CAD build for the part. Positions are in the model's coordinates, mm. Face numbers are marked on the shaded views. Give positions to 0.01 mm unless a question says otherwise; leave off trailing zeros. Loops run counter-clockwise (first coordinate to the right, second up) from the corner with the lowest first, then second, coordinate; pieces in that order, holes last.
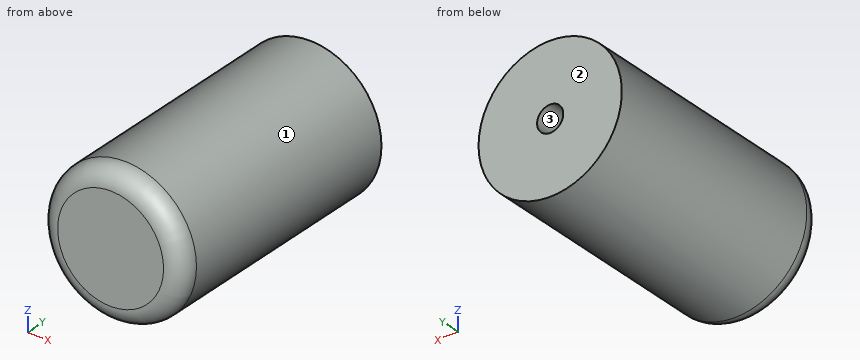
```python
from build123d import *

# Parameters (mm, degrees)
SKETCH1_R           = 11.5
BOSS_EXTRUDE1_DEPTH = 42
FILLET1_R           = 3
SKETCH3_R           = 2.1
CUT_EXTRUDE1_DEPTH  = 10


with BuildPart() as part:
    # Sketch1 → Boss-Extrude1 (new body)
    with BuildSketch(Plane(origin=(0, 0, 0), x_dir=(1, 0, 0), z_dir=(0, 1, 0))):
        Circle(SKETCH1_R)
    extrude(amount=BOSS_EXTRUDE1_DEPTH)

    # Fillet1
    fillet1_edges = [part.edges().sort_by_distance(p)[0] for p in [
        (-11.5, 0, 0),
    ]]
    fillet(fillet1_edges, radius=FILLET1_R)

    # Sketch3 → Cut-Extrude1 (cut)
    with BuildSketch(Plane(origin=(0, 42, 0), x_dir=(1, 0, 0), z_dir=(0, 1, 0))):
        Circle(SKETCH3_R)
    extrude(amount=-CUT_EXTRUDE1_DEPTH, mode=Mode.SUBTRACT)


solid = part.part
```
1. Drop flat-ended pins along their axis: pin 1 (5 mm diameter, centred on y = 30, z = 8.5, fed in from +X); pin 2 (1.5 mm diameter, centred on y = 10, z = -4.5, fed in from +X); pin 3 (3 mm diameter, centred on x = -6.5, y = 14.5, fed in from -Z). Give the stop position or say it passes through.
Responses:
pin 1: stops at x = 9.81
pin 2: stops at x = 10.87
pin 3: stops at z = -10.36
2. Saw through at C-C, the plane y = 34. List the corners of the cut face in (x, z), and give its area (3 significant figures).
Responses:
outline: circle Ø23 at (0, 0); hole circle Ø4.2 at (0, 0)
area: 402 mm2
3. Pull direction Z, two halves, no side cores. Call the marked faces 1, 2 and 3: released by +Z, released by -Z, zero draft, split by the parting line, or undercut.
Responses:
face 1: split by the parting line
face 2: zero draft
face 3: undercut
4. Saw through at A-A, the plane x = 0. List the corners of the cut face in (y, z), and give its area (3 significant figures).
Responses:
outline: (0, -8.5) arc R3 ccw to (3, -11.5) - (42, -11.5) - (42, -2.1) - (32, -2.1) - (32, 2.1) - (42, 2.1) - (42, 11.5) - (3, 11.5) arc R3 ccw to (0, 8.5) - close
area: 920 mm2
5. Probe line 1 along Z through (x, y) = (0, 38); line 2 along Y through (x, z) = (2.5, 8.25). List the from-to ranges inside material, lowest first.
Responses:
line 1: z = -11.5 to -2.1, 2.1 to 11.5
line 2: y = 0 to 42
6. Saw through at D-D, the plane y = 12.5. List the corners of the cut face in (x, z).
Responses:
outline: circle Ø23 at (0, 0)
7. Saw through at B-B, the plane z = 0. List the corners of the cut face in (x, y), and give its area (3 significant figures).
Responses:
outline: (-11.5, 3) arc R3 ccw to (-8.5, 0) - (8.5, 0) arc R3 ccw to (11.5, 3) - (11.5, 42) - (2.1, 42) - (2.1, 32) - (-2.1, 32) - (-2.1, 42) - (-11.5, 42) - close
area: 920 mm2
